Here's how the part is built. I have some questions about the finished solid (model axes, mm). A direction names the side the tool comes from. Give positions to 0.01 mm unless a question says otherwise; leave off trailing zeros. Loops run counter-clockwise (first coordinate to the right, second up) from the corner with the lowest first, then second, coordinate; pieces in that order, holes last. Notation, with made-up numbers: (53, 37.5) - (59, 37.5) arc R19 ccw to (59, 55.5) - close; hole circle Ø1 at (18.25, 27.25). An arc over 180 degrees is marked (long way). Use a Markdown table: item, result.
from build123d import *

# Parameters (mm, degrees)
SKETCH1_W                            = 125
SKETCH1_H                            = 120
TOP_BASE_DEPTH                       = 9
SKETCH5_R                            = 14
DRIVE_GEAR_EXTRUDE_CUT_DEPTH         = 6
SKETCH17_R                           = 19.75
INTERMEDIATE_GEAR_TOP_PART_CUT_DEPTH = 174.51080658
SKETCH8_R                            = 18.5
THUMB_EXTRUDE_CUT_DEPTH              = 174.51080658
SKETCH26_R                           = 1.5
STRING_HOLES_DEPTH                   = 174.51080658
THUMB_MOUNT_HOLES_R                  = 2.25
THUMB_MOUNT_HOLES_M4_DEPTH           = 174.51080658
FINGERS_MOUNT_HOLES_R                = 2.25
FINGERS_MOUNT_HOLES_M4_DEPTH         = 174.51080658
CONNECT_HOLES_POSITION_R             = 3.25
CONNECT_HOLES_M6_DEPTH               = 174.51080658
XL320_NUT_M4_DEPTH                   = 4


with BuildPart() as part:
    # Sketch1 → Top_Base (new body)
    with BuildSketch(Plane(origin=(0, 0, 0), x_dir=(1, 0, 0), z_dir=(0, 1, 0))):
        with Locations((62.5, 60)):
            Rectangle(SKETCH1_W, SKETCH1_H)
    extrude(amount=TOP_BASE_DEPTH)

    # Sketch5 → Drive_Gear_Extrude_Cut (cut)
    with BuildSketch(Plane(origin=(0, 9, 0), x_dir=(1, 0, 0), z_dir=(0, 1, 0))):
        with Locations(Location((34.75, 60, 0), (0, 0, 270))):
            Circle(SKETCH5_R)
    extrude(amount=-DRIVE_GEAR_EXTRUDE_CUT_DEPTH, mode=Mode.SUBTRACT)

    # Sketch17 → Intermediate_Gear_Top_Part_Cut (cut, through all)
    with BuildSketch(Plane(origin=(0, 9, 0), x_dir=(1, 0, 0), z_dir=(0, 1, 0))):
        with Locations(Location((63.146123438, 51.648511205, 0), (0, 0, 270))):
            Circle(SKETCH17_R)
    extrude(amount=-INTERMEDIATE_GEAR_TOP_PART_CUT_DEPTH, mode=Mode.SUBTRACT)

    # Sketch8 → Thumb_Extrude_Cut (cut, through all)
    with BuildSketch(Plane(origin=(0, 9, 0), x_dir=(1, 0, 0), z_dir=(0, 1, 0))):
        with Locations(Location((104.5, 60, 0), (0, 0, 270))):
            Circle(SKETCH8_R)
    extrude(amount=-THUMB_EXTRUDE_CUT_DEPTH, mode=Mode.SUBTRACT)

    # Sketch26 → String_Holes (cut, through all)
    with BuildSketch(Plane.XZ):
        with Locations(Location((37.25, -41, 0), (0, 0, 270))):
            Circle(SKETCH26_R)
        with Locations(Location((37.25, -79, 0), (0, 0, 90))):
            Circle(SKETCH26_R)
    extrude(amount=-STRING_HOLES_DEPTH, mode=Mode.SUBTRACT)

    # Thumb_Mount_Holes → Thumb_Mount_Holes_(M4) (cut, through all)
    with BuildSketch(Plane(origin=(0, 9, 0), x_dir=(1, 0, 0), z_dir=(0, 1, 0))):
        with Locations(Location((104.5, 113.5, 0), (0, 0, 270))):
            Circle(THUMB_MOUNT_HOLES_R)
        with Locations(Location((84, 104.5, 0), (0, 0, 270))):
            Circle(THUMB_MOUNT_HOLES_R)
        with Locations(Location((110.5, 36, 0), (0, 0, 270))):
            Circle(THUMB_MOUNT_HOLES_R)
        with Locations(Location((98.5, 36, 0), (0, 0, 90))):
            Circle(THUMB_MOUNT_HOLES_R)
    extrude(amount=-THUMB_MOUNT_HOLES_M4_DEPTH, mode=Mode.SUBTRACT)

    # Fingers_Mount_Holes → Fingers_Mount_Holes_(M4) (cut, through all)
    with BuildSketch(Plane(origin=(0, 9, 0), x_dir=(1, 0, 0), z_dir=(0, 1, 0))):
        with Locations(Location((74, 101, 0), (0, 0, 270))):
            Circle(FINGERS_MOUNT_HOLES_R)
        with Locations(Location((74, 19, 0), (0, 0, 90))):
            Circle(FINGERS_MOUNT_HOLES_R)
        with Locations(Location((10.75, 54, 0), (0, 0, 270))):
            Circle(FINGERS_MOUNT_HOLES_R)
        with Locations(Location((10.75, 66, 0), (0, 0, 90))):
            Circle(FINGERS_MOUNT_HOLES_R)
    extrude(amount=-FINGERS_MOUNT_HOLES_M4_DEPTH, mode=Mode.SUBTRACT)

    # Connect_Holes_Position → Connect_Holes_(M6) (cut, through all)
    with BuildSketch(Plane(origin=(0, 9, 0), x_dir=(1, 0, 0), z_dir=(0, 1, 0))):
        with Locations(Location((10, 110, 0), (0, 0, 270))):
            Circle(CONNECT_HOLES_POSITION_R)
        with Locations(Location((115, 10, 0), (0, 0, 270))):
            Circle(CONNECT_HOLES_POSITION_R)
        with Locations(Location((10, 10, 0), (0, 0, 270))):
            Circle(CONNECT_HOLES_POSITION_R)
    extrude(amount=-CONNECT_HOLES_M6_DEPTH, mode=Mode.SUBTRACT)

    # Sketch27 → XL320_Nut_(M4) (cut)
    with BuildSketch(Plane.XZ):
        Polygon((10.75, -49), (6.419872981, -51.5), (6.419872981, -56.5), (10.75, -59), (15.080127019, -56.5), (15.080127019, -51.5), align=None)
        Polygon((6.419872981, -63.5), (6.419872981, -68.5), (10.75, -71), (15.080127019, -68.5), (15.080127019, -63.5), (10.75, -61), align=None)
        Polygon((102.830127019, -38.5), (102.830127019, -33.5), (98.5, -31), (94.169872981, -33.5), (94.169872981, -38.5), (98.5, -41), align=None)
        Polygon((114.830127019, -33.5), (110.5, -31), (106.169872981, -33.5), (106.169872981, -38.5), (110.5, -41), (114.830127019, -38.5), align=None)
    extrude(amount=-XL320_NUT_M4_DEPTH, mode=Mode.SUBTRACT)


solid = part.part
(1) We'd pull the mould along Z, two halves only. Please class faces 4 (the face through (62, 0, -74)), 5 (the face through (8.55, 1.97, -69.73)), 6 (the face through (112.7, 1.97, -32.27)): pulls with the +Z half, pulls with the -Z half, needs draft (parallel to the pull), parting line crosses it, or undercut.
A:
| item | result |
|---|---|
| face 4 | needs draft |
| face 5 | undercut |
| face 6 | undercut |
(2) Suppose I cut it at C-C on x = 57. Write out the boundary of the cut face in (y, z).
A:
| item | result |
|---|---|
| outline | (0, -120) - (9, -120) - (9, -70.42) - (0, -70.42) - close; (0, -32.88) - (9, -32.88) - (9, 0) - (0, 0) - close |
(3) On a 3-axis mill with a long thin cutter (end or side, diameter ignored), from which of +Z, -Z, +X, -X, +Y, -Y can I reach the whole of each face in a straight line? I mean faces 1 (the face through (79.8, 4.56, -41.03)), 2 (the face through (21.468, 6.042, -64.425)), 3 (the face through (108.3, 1.97, -39.73)). Say none if no direction works.
A:
| item | result |
|---|---|
| face 1 | +Y, -Y |
| face 2 | +Y |
| face 3 | -Y |
(4) Suppose I cut it at B-B on y = 6. Count the separate pieces of the cut face and the enclosed holes in it, plus the area to 3 significant figures.
A:
| item | result |
|---|---|
| separate pieces | 1 |
| enclosed holes | 15 |
| area | 11,900 mm2 |
(5) Suppose I cut it at A-A on z = -10. Write out the boundary of the cut face in (x, y), plus the area to 3 significant figures.
A:
| item | result |
|---|---|
| outline | (0, 0) - (6.75, 0) - (6.75, 9) - (0, 9) - close; (13.25, 0) - (111.75, 0) - (111.75, 9) - (13.25, 9) - close; (118.25, 0) - (125, 0) - (125, 9) - (118.25, 9) - close |
| area | 1,010 mm2 |
(6) If I drill on line 1 (Z direction, x = 98.5, y = 7.1); line 2 (X direction, y = 4.25, z = -101); line 3 (Z direction, x = 37, y = 7.5), over which ranges is the centre line in solid material (lowest first)?
A:
| item | result |
|---|---|
| line 1 | -120 to -77.5, -42.5 to -38.25, -33.75 to 0 |
| line 2 | 0 to 71.75, 76.25 to 125 |
| line 3 | -120 to -80.48, -77.52 to -73.82, -46.18 to -42.48, -39.52 to 0 |
(7) Suppose I cut it at D-D on z = -100.5. Write out the boundary of the cut face in (x, y).
A:
| item | result |
|---|---|
| outline | (0, 0) - (71.81, 0) - (71.81, 9) - (0, 9) - close; (76.19, 0) - (125, 0) - (125, 9) - (76.19, 9) - close |
